```python
from build123d import *

# Parameters (mm, degrees)
F0_R     = 10.16
F1_DEPTH = 15.7734
F2_DEPTH = 40.2336
F3_R     = 3.302


with BuildPart() as f1:
    # F0 (on Front) → F1 (new body)
    with BuildSketch(Plane.XZ):
        with BuildLine():
            ThreePointArc((10.077445, 26.73903), (23.499932, 16.256808), (28.575, 0))
            ThreePointArc((28.575, 0), (23.499932, -16.256808), (10.077445, -26.73903))
            Line((10.077445, -26.73903), (53.975, -18.741507))
            ThreePointArc((53.975, -18.741507), (69.610559, 0), (53.975, 18.741507))
            Line((53.975, 18.741507), (10.077445, 26.73903))
        make_face()
        with Locations((53.975, 0)):
            Circle(F0_R, mode=Mode.SUBTRACT)
    extrude(amount=F1_DEPTH)

    # F0 (on Front) → F2 (join)
    with BuildSketch(Plane.XZ):
        with BuildLine():
            ThreePointArc((10.077445, -26.73903), (23.499932, -16.256808), (28.575, 0))
            ThreePointArc((28.575, 0), (23.499932, 16.256808), (10.077445, 26.73903))
            ThreePointArc((10.077445, 26.73903), (-28.575, 0), (10.077445, -26.73903))
        make_face()
        with BuildLine():
            ThreePointArc((13.447765, -4.826), (-14.2875, 0), (13.447765, 4.826))
            Line((13.447765, 4.826), (18.5293, 4.826))
            Line((18.5293, 4.826), (18.5293, -4.826))
            Line((18.5293, -4.826), (13.447765, -4.826))
        make_face(mode=Mode.SUBTRACT)
    extrude(amount=F2_DEPTH)

    # F3
    f3_edges = [f1.edges().sort_by_distance(p)[0] for p in [
        (-10.077445, -40.2336, 26.73903),
    ]]
    fillet(f3_edges, radius=F3_R)


solid = f1.part
```
Geometry: final body of the model. Coordinates: model frame, mm. A direction names the side the tool comes from. Coordinates: 2 decimals unless noted, no trailing zeros. Order: outer loops, then holes, each group sorted by start corner. A loop starts at its lowest first (then second) coordinate and runs counter-clockwise, first axis right, second up. Notation, with made-up numbers: (15, -18.5) -> (71, -18.5) arc R26 cw to (71, -2.5) -> close; hole circle Ø5 at (-24, -23). An arc over 180 degrees is marked (long way). Write item = value, one per line.
(1) Line query: line 1 (Z direction, x = 0, y = -25) (1 decimal); line 2 (X direction, y = -34, z = 0) (1 decimal); line 3 (X direction, y = -10, z = -4). Output: solid intervals per line, ascending.
Solved:
line_1 = -28.6 to -14.3, 14.3 to 28.6
line_2 = -28.6 to -14.3, 18.5 to 28.6
line_3 = -28.29 to -13.72, 18.53 to 44.64, 63.31 to 69.19
(2) Access query for faces 1 (the flat face through (11, -40.234, -11)), 2 (the flat face through (18.529, -20, 0)). Directions: +Z, -Z, +X, -X, +Y, -Y. A direction counts if a zero-diameter tool reaches every point of the face in a straight line with its end or side. Return the directions, or none.
Solved:
face_1 = +Z, -Z, +X, -X, -Y
face_2 = +Y, -Y
(3) Cut plane A-A on y = -5. Count the separate pieces of the cut face and the enclosed holes in it, plus the area to 3 significant figures.
Solved:
separate_pieces = 1
enclosed_holes = 2
area = 3,270 mm²
(4) Pull-direction query (X, two-part tool) for faces 3 (the flat face through (31.7, -7.8, -22.8)), 4 (the flat face through (16, -20, -4.826)), 5 (the flat face through (20, 0, 0)); classes: pulls with the +X half, pulls with the -X half, needs draft (parallel to the pull), parting line crosses it, or undercut.
Solved:
face_3 = pulls with the +X half
face_4 = undercut
face_5 = needs draft
(5) Cut plane B-B on x = 49. Return loops of the section in (y, z), plus the area to 3 significant figures.
Solved:
outline = (-15.77, -19.65) -> (0, -19.65) -> (0, -8.86) -> (-15.77, -8.86) -> close; (-15.77, 8.86) -> (0, 8.86) -> (0, 19.65) -> (-15.77, 19.65) -> close
area = 340 mm²
(6) Pin query (flat end, axial travel): pin 1 Ø6 at (x, y) = (41.5, -18.5) entering from +Z; pin 2 Ø1.5 at (x, y) = (17, -17.5) entering from +Z; pin 3 Ø5.5 at (x, y) = (16.5, -23) entering from -Z; pin 4 Ø17 at (x, z) = (0, 0) entering from -Y. Return the tip coordinate at first contact, or that it passes through.
Solved:
pin_1 = 21.24
pin_2 = 23.5
pin_3 = -25.05
pin_4 = through
